Geometry: final body of the model. Coordinates: model frame, mm. Coordinates: 2 decimals unless noted, no trailing zeros. Write each loop counter-clockwise with the first axis right and the second up, starting at its lowest first coordinate (ties: lowest second). Pieces come first, ordered by that corner, then holes. Notation, with made-up numbers: (9.25, 2.5) -> (17.25, 2.5) arc R26 cw to (17.25, 17.5) -> close; hole circle Ø1 at (4, -31). An arc over 180 degrees is marked (long way). One line per item, written item: value.
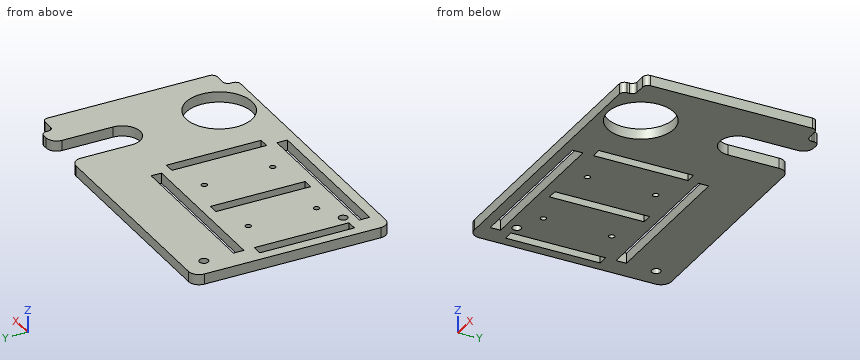
```python
from build123d import *
from OCP.BRepFilletAPI import BRepFilletAPI_MakeFillet

# Parameters (mm, degrees)
SKETCH1_R                   = 20.2311
BOSS_EXTRUDE1_DEPTH         = 6.35
FILLET1_R1                  = 6.35
FILLET1_R2                  = 3.175
TAP_DRILL_FOR_8_32_TAP3_D   = 3.4544
TAP_DRILL_FOR_1_4_28_TAP1_D = 5.4102
SKETCH13_W                  = 95.25
SKETCH13_H                  = 6.35
SKETCH13_W_2                = 6.35
SKETCH13_H_2                = 57.927875
CUT_EXTRUDE1_DEPTH          = 136.524699219


with BuildPart() as part:
    # Sketch1 → Boss-Extrude1 (new body)
    with BuildSketch(Plane.XY):
        with BuildLine():
            Line((-114.3, 72.540551407), (28.4099, 72.540551407))
            Line((28.4099, 72.540551407), (28.4099, 35.1155))
            ThreePointArc((28.4099, 35.1155), (39.37, 24.1554), (50.3301, 35.1155))
            Line((50.3301, 35.1155), (50.3301, 72.540551407))
            Line((50.3301, 72.540551407), (62.738, 72.540551407))
            Line((62.738, 72.540551407), (62.738, 64.920551407))
            Line((62.738, 64.920551407), (75.438, 64.920551407))
            Line((75.438, 64.920551407), (75.438, -40.3939375))
            Line((75.438, -40.3939375), (62.738, -40.3939375))
            Line((62.738, -40.3939375), (62.738, -48.0139375))
            Line((62.738, -48.0139375), (-114.3, -48.0139375))
            Line((-114.3, -48.0139375), (-114.3, 72.540551407))
        make_face()
        with Locations((39.37, -24.152515463)):
            Circle(SKETCH1_R, mode=Mode.SUBTRACT)
    extrude(amount=BOSS_EXTRUDE1_DEPTH)

    # Fillet1: one fillet with a radius per group of edges: ONE call of the kernel's fillet builder (fillet() takes one radius for all edges)
    fillet1_edges_1 = [part.edges().sort_by_distance(p)[0] for p in [
        (50.3301, 72.540551407, 3.175),
        (28.4099, 72.540551407, 3.175),
        (-114.3, 72.540551407, 3.175),
        (-114.3, -48.0139375, 3.175),
    ]]
    fillet1_edges_2 = [part.edges().sort_by_distance(p)[0] for p in [
        (62.738, 64.920551407, 3.175),
        (75.438, 64.920551407, 3.175),
        (62.738, 72.540551407, 3.175),
        (62.738, -48.0139375, 3.175),
        (62.738, -40.3939375, 3.175),
        (75.438, -40.3939375, 3.175),
    ]]
    fillet1 = BRepFilletAPI_MakeFillet(part.part.solid().wrapped)
    for e in fillet1_edges_1:
        fillet1.Add(FILLET1_R1, e.wrapped)
    for e in fillet1_edges_2:
        fillet1.Add(FILLET1_R2, e.wrapped)
    add(Compound.cast(fillet1.Shape()), mode=Mode.REPLACE)

    # Tap Drill for #8-32 Tap3 (through all)
    with Locations(Plane(origin=(-189.82086846, 75.287041891, 6.35), x_dir=(0, -1, 0), z_dir=(0, 0, 1))):
        with Locations((54.400304391, 110.44586846), (96.173779391, 110.44586846), (96.173779391, 161.24586846), (54.400304391, 161.24586846)):
            Hole(TAP_DRILL_FOR_8_32_TAP3_D / 2)

    # Tap Drill for 1/4-28 Tap1 (through all)
    with Locations(Plane(origin=(-189.82086846, 75.287041891, 6.35), x_dir=(0, 1, 0), z_dir=(0, 0, 1))):
        with Locations((-15.446490484, -88.22086846), (-104.052541891, -94.57086846)):
            Hole(TAP_DRILL_FOR_1_4_28_TAP1_D / 2)

    # Sketch13 → Cut-Extrude1 (cut, through all)
    with BuildSketch(Plane.XY.offset(6.35)):
        with Locations((-53.975, -38.4889375)):
            Rectangle(SKETCH13_W, SKETCH13_H)
        with Locations((-53.975, 0)):
            Rectangle(SKETCH13_W_2, SKETCH13_H_2)
        with Locations((-3.175, 0)):
            Rectangle(SKETCH13_W_2, SKETCH13_H_2)
        with Locations((-53.975, 38.4889375)):
            Rectangle(SKETCH13_W, SKETCH13_H)
        with Locations((-104.775, 0)):
            Rectangle(SKETCH13_W_2, SKETCH13_H_2)
    extrude(amount=-CUT_EXTRUDE1_DEPTH, mode=Mode.SUBTRACT)


solid = part.part
```
(1) Section A-A (x = -47). Return the cut outline in (y, z).
Responses:
outline: (-48.01, 0) -> (-41.66, 0) -> (-41.66, 6.35) -> (-48.01, 6.35) -> close; (-35.31, 0) -> (35.31, 0) -> (35.31, 6.35) -> (-35.31, 6.35) -> close; (41.66, 0) -> (72.54, 0) -> (72.54, 6.35) -> (41.66, 6.35) -> close
(2) Line query: line 1 (Y direction, x = -41.5, z = 5.25); line 2 (X direction, y = 18, z = 2.75); line 3 (Y direction, x = -95.25, z = 3). Output: solid intervals per line, ascending. Write a range as [from, to].
Responses:
line 1: y = [-48.01, -41.66], [-35.31, 35.31], [41.66, 72.54]
line 2: x = [-114.3, -107.95], [-101.6, -57.15], [-50.8, -6.35], [0, 75.44]
line 3: y = [-48.01, -41.66], [-35.31, -31.47], [-26.06, 35.31], [41.66, 72.54]
(3) First-contact query: pin 1 (1 mm diameter, centred on y = -44.5, z = 2, fed in from +X). Flat tip, straight axial feed; report the tip coordinate or a pass-through.
Responses:
pin 1: stops at x = 62.74
(4) Section D-D (x = -95.25). Return the cut outline in (y, z), then the cut area to 3 significant figures.
Responses:
outline: (-48.01, 0) -> (-41.66, 0) -> (-41.66, 6.35) -> (-48.01, 6.35) -> close; (-35.31, 0) -> (-31.47, 0) -> (-31.47, 6.35) -> (-35.31, 6.35) -> close; (-26.06, 0) -> (35.31, 0) -> (35.31, 6.35) -> (-26.06, 6.35) -> close; (41.66, 0) -> (72.54, 0) -> (72.54, 6.35) -> (41.66, 6.35) -> close
area: 651 mm2
(5) Section B-B (x = 39.37). Return the cut outline in (y, z), then the cut area to 3 significant figures.
Responses:
outline: (-48.01, 0) -> (-44.38, 0) -> (-44.38, 6.35) -> (-48.01, 6.35) -> close; (-3.92, 0) -> (24.16, 0) -> (24.16, 6.35) -> (-3.92, 6.35) -> close
area: 201 mm2
(6) Section C-C (y = 26.5). Return the cut outline in (x, z).
Responses:
outline: (-114.3, 0) -> (-107.95, 0) -> (-107.95, 6.35) -> (-114.3, 6.35) -> close; (-101.6, 0) -> (-57.15, 0) -> (-57.15, 6.35) -> (-101.6, 6.35) -> close; (-50.8, 0) -> (-6.35, 0) -> (-6.35, 6.35) -> (-50.8, 6.35) -> close; (0, 0) -> (32.6, 0) -> (32.6, 6.35) -> (0, 6.35) -> close; (46.14, 0) -> (75.44, 0) -> (75.44, 6.35) -> (46.14, 6.35) -> close
